For this review, take the finished solid that the model builds, in its own axes (mm). A direction names the side the tool comes from. Round coordinates to 2 decimals unless told otherwise and drop trailing zeros. Order: outer loops, then holes, each group sorted by start corner. A loop starts at its lowest first (then second) coordinate and runs counter-clockwise, first axis right, second up. Notation, with made-up numbers: (-6.5, 61) -> (26.5, 61) arc R32 cw to (26.5, 100) -> close; hole circle Ø4 at (58.25, -36.75). An arc over 180 degrees is marked (long way). Put each result on its own line as item: value. Start each with the question number.
```python
from build123d import *

# Parameters (mm, degrees)
EXTRUDE_1_DEPTH     = 8
CUT_EXTRUDE_1_DEPTH = 5
EXTRUDE_START       = 17
SKETCH_3_R          = 15
EXTRUDE_2_DEPTH     = 17
EXTRUDE_3_DEPTH     = 10


with BuildPart() as part:
    # 스케치1 → 보스-돌출1 (new body)
    with BuildSketch(Plane.XY):
        with BuildLine():
            Line((-15, 15), (-15, -15))
            ThreePointArc((-15, -15), (0, -30), (15, -15))
            Line((15, -15), (15, 15))
            ThreePointArc((15, 15), (0, 30), (-15, 15))
        make_face()
    extrude(amount=EXTRUDE_1_DEPTH)

    # 스케치2 → 컷-돌출1 (cut)
    with BuildSketch(Plane.XY.offset(8)):
        Polygon((0, 19.942281197), (-4.700388737, 16.527248881), (-2.905, 11.001610521), (2.905, 11.001610521), (4.700388737, 16.527248881), align=None)
    extrude(amount=-CUT_EXTRUDE_1_DEPTH, mode=Mode.SUBTRACT)

    # 스케치3 → 보스-돌출2 (add)
    with BuildSketch(Plane(origin=(0, 0, 0), x_dir=(-1, 0, 0), z_dir=(0, 0, -1)).offset(EXTRUDE_START)):
        with Locations((0, -15)):
            Circle(SKETCH_3_R)
    extrude(amount=-EXTRUDE_2_DEPTH)

    # 스케치4 → 보스-돌출3 (add)
    with BuildSketch(Plane(origin=(0, 0, -17), x_dir=(-1, 0, 0), z_dir=(0, 0, -1))):
        Polygon((0, -8.819660113), (-5.877852523, -13.090169944), (-3.63271264, -20), (3.63271264, -20), (5.877852523, -13.090169944), align=None)
    extrude(amount=EXTRUDE_3_DEPTH)


solid = part.part
```
Item 1: Tool access review of faces 4 (the face through (-2.317, 18.259, 5.535)), 5 (the face through (0, -20, -22)), 6 (the face through (4.77, -16.5, -21.93)): name each direction out of +Z, -Z, +X, -X, +Y, -Y from which nothing blocks a thin tool from reaching the whole face with its end or side.
Item 2: Mouldability with a two-part tool opening along Y and no side actions: class faces 1 (the face through (-4.74, -16.59, -21.93)), 2 (the face through (-15, 0, 4)), 3 (the face through (3.79, 13.73, 5.54)) as +Y half, -Y half, draft (parallel to the pull), parting line (faces both ways), or undercut.
Item 3: Insertion check: pin 1 Ø3.5 at (x, z) = (1.5, -20) entering from -Y; pin 2 Ø4.5 at (x, y) = (-0.5, 14) entering from +Z; pin 3 Ø1.5 at (x, z) = (-4, -22) entering from +Y. Each pin has a flat end and moves straight along its axis. Give the tip position at first contact, or say it passes through.
Item 4: Consider section B-B, the plane z = -3.5. Write out the cut boundary in (x, y), plus the area to 3 significant figures.
Item 5: For L1, parallel to Z at x = -2, y = 23.5; L2, parallel to Z at x = -8, y = -27; L3, parallel to Y at x = -0.5, z = -1.5, list the stretches that pass through material, from the lowest coordinate up.
Item 6: Consider section D-D, the plane z = 1. Write out the cut boundary in (x, y).
Item 7: Consider section A-A, the plane x = -1. Write out the cut boundary in (y, z), plus the area to 3 significant figures.
Item 8: Consider section C-C, the plane y = -12. Write out the cut boundary in (x, z).
Evaluation:
1. face 4: +Z
1. face 5: -Z, +X, -X, -Y
1. face 6: -Z, +X, -Y
2. face 1: -Y half
2. face 2: draft
2. face 3: undercut
3. pin 1: stops at y = -20
3. pin 2: stops at z = 3
3. pin 3: stops at y = -11.18
4. outline: circle Ø30 at (0, -15)
4. area: 707 mm^2
5. L1: z = 0 to 8
5. L2: z = -17 to 8
5. L3: y = -29.99 to -0.01
6. outline: (-15, -15) arc R15 ccw to (15, -15) -> (15, 15) arc R15 ccw to (-15, 15) -> close
7. outline: (-29.97, -17) -> (-20, -17) -> (-20, -27) -> (-9.55, -27) -> (-9.55, -17) -> (-0.03, -17) -> (-0.03, 0) -> (29.97, 0) -> (29.97, 8) -> (19.22, 8) -> (19.22, 3) -> (11, 3) -> (11, 8) -> (-29.97, 8) -> close
7. area: 1,050 mm^2
8. outline: (-15, 0) -> (-14.7, 0) -> (-14.7, -17) -> (-4.38, -17) -> (-4.38, -27) -> (4.38, -27) -> (4.38, -17) -> (14.7, -17) -> (14.7, 0) -> (15, 0) -> (15, 8) -> (-15, 8) -> close
